Geometry: final body of the model. Coordinates: model frame, mm. A direction names the side the tool comes from. Round coordinates to 2 decimals unless told otherwise and drop trailing zeros. Answer as a JSON object with one key per item and string values. Group by question number.
Item 1: First-contact query: pin 1 (3 mm diameter, centred on x = -139, z = -3, fed in from -Y). Flat tip, straight axial feed; report the tip coordinate or a pass-through.
Item 2: Line query: line 1 (Y direction, x = 157, z = -10.5); line 2 (Y direction, x = 56, z = -7); line 3 (Z direction, x = -59.5, y = -8.5). Output: solid intervals per line, ascending.
Item 3: Reachability of faces 1 (the face through (68, 0, -6.35)), 2 (the face through (-3, -31.75, -9)) from +Z, -Z, +X, -X, +Y, -Y: full face, straight path, thin tool, end or side. Return the list, or none.
Item 4: Section A-A (z = -8.5). Count the separate pieces of the cut face and the enclosed holes in it, plus the area to 3 significant figures.
```python
from build123d import *

# Parameters (mm, degrees)
F0_W     = 457.2
F0_H     = 63.5
F1_DEPTH = 12.7
F2_W     = 304.8
F2_H     = 50.8
F3_DEPTH = 6.35
F3_TAPER = 20
F4_R     = 5.08
F5_R     = 2.54
F6_DEPTH = 12.7010001
F6_TAPER = -30


with BuildPart() as f1:
    # F0 (on Top) → F1 (new body)
    with BuildSketch(Plane.XY):
        Rectangle(F0_W, F0_H)
    extrude(amount=-F1_DEPTH)

    # F2 (on face) → F3 (cut)
    with BuildSketch(Plane.XY):
        with Locations((69.85, 0)):
            Rectangle(F2_W, F2_H)
    extrude(amount=-F3_DEPTH, taper=F3_TAPER, mode=Mode.SUBTRACT)

    # F4
    f4_edges = [f1.edges().sort_by_distance(p)[0] for p in [
        (0, 31.75, 0),
        (228.6, 0, 0),
        (228.6, 31.75, -6.35),
        (228.6, -31.75, -6.35),
        (-228.6, 31.75, -6.35),
        (-228.6, 0, 0),
        (0, -31.75, 0),
        (-228.6, -31.75, -6.35),
    ]]
    fillet(f4_edges, radius=F4_R)

    # F5 (on face) → F6 (cut, through all)
    with BuildSketch(Plane(origin=(0, 0, -12.7), x_dir=(1, 0, 0), z_dir=(0, 0, -1))):
        with Locations((207.2387890124, -10.3887890124)):
            Circle(F5_R)
        with Locations((207.2387890124, 10.3887890124)):
            Circle(F5_R)
        with Locations((181.8387890124, -10.3887890124)):
            Circle(F5_R)
        with Locations((181.8387890124, 10.3887890124)):
            Circle(F5_R)
        with Locations((156.4387890124, -10.3887890124)):
            Circle(F5_R)
        with Locations((156.4387890124, 10.3887890124)):
            Circle(F5_R)
        with Locations((131.0387890124, -10.3887890124)):
            Circle(F5_R)
        with Locations((131.0387890124, 10.3887890124)):
            Circle(F5_R)
        with Locations((105.6387890124, -10.3887890124)):
            Circle(F5_R)
        with Locations((105.6387890124, 10.3887890124)):
            Circle(F5_R)
        with Locations((80.2387890124, -10.3887890124)):
            Circle(F5_R)
        with Locations((80.2387890124, 10.3887890124)):
            Circle(F5_R)
        with Locations((54.8387890124, -10.3887890124)):
            Circle(F5_R)
        with Locations((54.8387890124, 10.3887890124)):
            Circle(F5_R)
        with Locations((29.4387890124, -10.3887890124)):
            Circle(F5_R)
        with Locations((29.4387890124, 10.3887890124)):
            Circle(F5_R)
        with Locations((4.0387890124, -10.3887890124)):
            Circle(F5_R)
        with Locations((4.0387890124, 10.3887890124)):
            Circle(F5_R)
        with Locations((-21.3612109876, -10.3887890124)):
            Circle(F5_R)
        with Locations((-21.3612109876, 10.3887890124)):
            Circle(F5_R)
    extrude(amount=-F6_DEPTH, taper=F6_TAPER, mode=Mode.SUBTRACT)


solid = f1.part
```
Values:
{
 "1": {"pin 1": "stops at y = -31.72"},
 "2": {"line 1": "y = -31.75 to -14.16, -6.62 to 6.62, 14.16 to 31.75", "line 2": "y = -31.75 to -16.1, -4.67 to 4.67, 16.1 to 31.75", "line 3": "z = -12.7 to -6.35"},
 "3": {"face 1": "+Z", "face 2": "+Z, -Z, +X, -X, -Y"},
 "4": {"separate pieces": "1", "enclosed holes": "20", "area": "27,500 mm^2"}
}
